from build123d import *

# Parameters (mm, degrees)
EXTRUDE_1_DEPTH     = 20
CHAMFER_1_SIZE      = 2
SKETCH_2_R          = 4
EXTRUDE_2_DEPTH     = 3.5
SKETCH_3_R          = 2.1
CUT_EXTRUDE_1_DEPTH = 26.865227623
CHAMFER_2_SIZE      = 0.2
CHAMFER_3_SIZE      = 0.5


with BuildPart() as part:
    # 草图1 → 凸台-拉伸1 (new body)
    with BuildSketch(Plane(origin=(0, 0, 0), x_dir=(1, 0, 0), z_dir=(0, 1, 0))):
        Polygon((-7, 12.6), (0, 12.6), (0, -12.6), (-7, -12.6), (-7, -7.6), (-3, -7.6), (-3, 7.6), (-7, 7.6), align=None)
    extrude(amount=EXTRUDE_1_DEPTH)

    # 倒角1
    chamfer_1_edges = [part.edges().sort_by_distance(p)[0] for p in [
        (0, 10, -12.6),
        (0, 10, 12.6),
    ]]
    chamfer(chamfer_1_edges, length=CHAMFER_1_SIZE)

    # 草图2 → 凸台-拉伸2 (add)
    with BuildSketch(Plane(origin=(0, 0, 0), x_dir=(0, 0, -1), z_dir=(1, 0, 0))):
        with Locations(Location((0, 10, 0), (0, 0, 180))):
            Circle(SKETCH_2_R)
    extrude(amount=EXTRUDE_2_DEPTH)

    # 草图3 → 切除-拉伸1 (cut, through all)
    with BuildSketch(Plane(origin=(3.5, 0, 0), x_dir=(0, 0, -1), z_dir=(1, 0, 0))):
        with Locations((0, 10)):
            Circle(SKETCH_3_R)
    extrude(amount=-CUT_EXTRUDE_1_DEPTH, mode=Mode.SUBTRACT)

    # 倒角2
    chamfer_2_edges = [part.edges().sort_by_distance(p)[0] for p in [
        (3.5, 10, 2.1),
    ]]
    chamfer(chamfer_2_edges, length=CHAMFER_2_SIZE)

    # 倒角3
    chamfer_3_edges = [part.edges().sort_by_distance(p)[0] for p in [
        (-7, 10, 7.6),
        (-7, 10, -7.6),
    ]]
    chamfer(chamfer_3_edges, length=CHAMFER_3_SIZE)


solid = part.part
Geometry: final body of the model. Coordinates: model frame, mm. A direction names the side the tool comes from. Coordinates: 2 decimals unless noted, no trailing zeros. Order: outer loops, then holes, each group sorted by start corner. A loop starts at its lowest first (then second) coordinate and runs counter-clockwise, first axis right, second up. Notation, with made-up numbers: M 8.25,60.5 L 24.25,60.5 A12 cw 24.25,72.5 Z; hole C -27.75,8.25 d1. An arc over 180 degrees is marked long. One line per question, with ' | ' between items. Start each with the question number.
Item 1: Cut plane B-B, the plane x = -5.75. Return the cut outline in (y, z).
Item 2: Draft query along Z for faces 1 (the flat face through (-1, 9.9, 11.6)), 2 (the flat face through (-1, 9.9, -11.6)), 3 (the flat face through (-2.7, 20, -0.2)), 4 (the flat face through (-5, 10, 7.6)). Return one class per face: released by +Z, released by -Z, zero draft, split by the parting line, or undercut.
Item 3: Pin query (flat end, axial travel): pin 1 Ø7.5 at (y, z) = (9.5, -3.5) entering from -X; pin 2 Ø2 at (y, z) = (5.5, -10) entering from +X. Return the tip coordinate at first contact, or that it passes through.
Item 4: Cut plane D-D, the plane y = 3.5. Return the cut outline in (x, z).
Item 5: Cut plane A-A, the plane z = 0. Return the cut outline in (x, y), then the cut area to 3 significant figures.
Item 6: Set-up query: faces 5 (the flat face through (-5, 10, -7.6)), 6 (the flat face through (-4, 10, 12.6)), 7 (the flat face through (0, 5, 0)). Return all of +Z, -Z, +X, -X, +Y, -Y with unobstructed straight access to the full face (end or side cutting, diameter ignored); none if empty.
Item 7: Cut plane C-C, the plane y = 10. Return the cut outline in (x, z), then the cut area to 3 significant figures.
Item 8: Ray query, probe 1 along Y at (x, z) = (0.75, 0); probe 2 along Z at (x, y) = (-6.25, 9.5); probe 3 along Y at (x, z) = (-0.25, 0). Return the intervals inside material, ascending. Write a range as [from, to].
A:
1) outline: M 0,-12.6 L 20,-12.6 L 20,-7.6 L 0,-7.6 Z; M 0,7.6 L 20,7.6 L 20,12.6 L 0,12.6 Z
2) face 1: released by +Z | face 2: released by -Z | face 3: zero draft | face 4: undercut
3) pin 1: stops at x = -3 | pin 2: stops at x = 0
4) outline: M -7,-12.6 L -2,-12.6 L 0,-10.6 L 0,10.6 L -2,12.6 L -7,12.6 L -7,8.1 L -6.5,7.6 L -3,7.6 L -3,-7.6 L -6.5,-7.6 L -7,-8.1 Z
5) outline: M -3,0 L 0,0 L 0,6 L 3.5,6 L 3.5,7.7 L 3.3,7.9 L -3,7.9 Z; M -3,12.1 L 3.3,12.1 L 3.5,12.3 L 3.5,14 L 0,14 L 0,20 L -3,20 Z | area: 60.7 mm2
6) face 5: -X, +Y, -Y | face 6: +Z, +X, -X, +Y, -Y | face 7: +X
7) outline: M -7,-12.6 L -2,-12.6 L 0,-10.6 L 0,-4 L 3.5,-4 L 3.5,-2.3 L 3.3,-2.1 L -3,-2.1 L -3,-7.6 L -6.5,-7.6 L -7,-8.1 Z; M -7,8.1 L -6.5,7.6 L -3,7.6 L -3,2.1 L 3.3,2.1 L 3.5,2.3 L 3.5,4 L 0,4 L 0,10.6 L -2,12.6 L -7,12.6 Z | area: 112 mm2
8) probe 1: y = [6, 7.9], [12.1, 14] | probe 2: z = [-12.6, -7.6], [7.6, 12.6] | probe 3: y = [0, 7.9], [12.1, 20]
